```python
from build123d import *

# Parameters (mm, degrees)
F1_DEPTH = 20
F2_R     = 4
F3_DEPTH = 40.1223203436
F6_D     = 6.6


# Not quite as in the source:
# - a pattern or mirror of a feature is missing from the dataset's text; its kind, count and spacing are read off the source's solid


with BuildPart() as f1:
    # F0 (on Front) → F1 (new body, symmetric)
    with BuildSketch(Plane.XZ):
        with BuildLine():
            Line((-17.9289321881, 0), (0, 0))
            Line((0, 0), (17.9289321881, 0))
            ThreePointArc((17.9289321881, 0), (19.84234935, 0.3806023374), (21.4644660941, 1.4644660941))
            Line((21.4644660941, 1.4644660941), (55, 35))
            ThreePointArc((55, 35), (55, 39.2426406871), (50.7573593129, 39.2426406871))
            Line((50.7573593129, 39.2426406871), (18.9791847198, 7.4644660941))
            ThreePointArc((18.9791847198, 7.4644660941), (17.3570679757, 6.3806023374), (15.4436508139, 6))
            Line((15.4436508139, 6), (0, 6))
            Line((0, 6), (-15.4436508139, 6))
            ThreePointArc((-15.4436508139, 6), (-17.3570679757, 6.3806023374), (-18.9791847198, 7.4644660941))
            Line((-18.9791847198, 7.4644660941), (-50.7573593129, 39.2426406871))
            ThreePointArc((-50.7573593129, 39.2426406871), (-55, 39.2426406871), (-55, 35))
            Line((-55, 35), (-21.4644660941, 1.4644660941))
            ThreePointArc((-21.4644660941, 1.4644660941), (-19.84234935, 0.3806023374), (-17.9289321881, 0))
        make_face()
    extrude(amount=F1_DEPTH, both=True)

    # F2 (on Top) → F3 (cut, through all)
    with BuildSketch(Plane.XY):
        Circle(F2_R)
    extrude(amount=F3_DEPTH, mode=Mode.SUBTRACT)

    # F6 (through all)
    with Locations(Plane(origin=(10, 0, -10), x_dir=(0, 1, 0), z_dir=(0.7071067812, 0, -0.7071067812))):
        with Locations((0, 53.1789772213)):
            f6 = Hole(F6_D / 2)

    # F6_copies: F6 across plane
    add(f6.mirror(Plane(origin=(0, 0, 0), x_dir=(0, 0, -1), z_dir=(-1, 0, 0))), mode=Mode.SUBTRACT)


solid = f1.part
```
Build history of the part. All positions in model axes, mm. A direction names the side the tool comes from. Round coordinates to 2 decimals unless told otherwise and drop trailing zeros. Order: outer loops, then holes, each group sorted by start corner. A loop starts at its lowest first (then second) coordinate and runs counter-clockwise, first axis right, second up. Notation, with made-up numbers: (-10.5, 51.5) - (23.5, 51.5) arc R5 cw to (23.5, 57.5) - close; hole circle Ø7 at (-12.5, -31.5). An arc over 180 degrees is marked (long way). Use a Markdown table: item, result.
1) Saw through at B-B on y = 0. Write the cut outline in (x, z), and give its area (3 significant figures).
Recorded:
| item | result |
|---|---|
| outline | (-55, 35) - (-49.94, 29.94) - (-45.69, 34.18) - (-50.76, 39.24) arc R3 ccw to start; (-45.27, 25.27) - (-21.46, 1.46) arc R5 ccw to (-17.93, 0) - (-4, 0) - (-4, 6) - (-15.44, 6) arc R5 cw to (-18.98, 7.46) - (-41.03, 29.51) - close; (4, 0) - (17.93, 0) arc R5 ccw to (21.46, 1.46) - (45.27, 25.27) - (41.03, 29.51) - (18.98, 7.46) arc R5 cw to (15.44, 6) - (4, 6) - close; (45.69, 34.18) - (49.94, 29.94) - (55, 35) arc R3 ccw to (50.76, 39.24) - close |
| area | 705 mm² |
2) Saw through at C-C on y = -12. Write the cut outline in (x, z).
Recorded:
| item | result |
|---|---|
| outline | (-55, 35) - (-21.46, 1.46) arc R5 ccw to (-17.93, 0) - (17.93, 0) arc R5 ccw to (21.46, 1.46) - (55, 35) arc R3 ccw to (50.76, 39.24) - (18.98, 7.46) arc R5 cw to (15.44, 6) - (-15.44, 6) arc R5 cw to (-18.98, 7.46) - (-50.76, 39.24) arc R3 ccw to start |
3) Pull direction X, two halves, no side cores. Call faces 3 (the face through (-54.95, -0.28, 39.29)), 4 (the face through (-19.87, -0.28, 0.39)), 5 (the face through (-4.2, -0.3, 0)): pulls with the +X half, pulls with the -X half, needs draft (parallel to the pull), parting line crosses it, or undercut.
Recorded:
| item | result |
|---|---|
| face 3 | undercut |
| face 4 | pulls with the -X half |
| face 5 | needs draft |
4) Wall check: L1, parallel to Y at x = 0, z = 3.75; L2, parallel to Z at x = -9.5, y = -12; L3, parallel to X at y = 14, z = 17.5. Give the ranges that are in metal, low to high.
Recorded:
| item | result |
|---|---|
| L1 | y = -20 to -4, 4 to 20 |
| L2 | z = 0 to 6 |
| L3 | x = -37.5 to -29.01, 29.01 to 37.5 |
5) Flat gauge pins, fed straight in: pin 1 Ø1.5 at (x, z) = (-42.5, 32) entering from +Y; pin 2 Ø6.5 at (x, y) = (0, 0) entering from +Z; pin 3 Ø1.5 at (x, y) = (20.5, 7) entering from +Z; pin 4 Ø4 at (y, z) = (5, 31) entering from -X. Where does each tip first touch, or does it go through?
Recorded:
| item | result |
|---|---|
| pin 1 | stops at y = 20 |
| pin 2 | passes through |
| pin 3 | stops at z = 9.74 |
| pin 4 | stops at x = -53 |
6) Tool access for faces 1 (the face through (17.4, -0.3, 6.4)), 2 (the face through (19.82, -0.28, 0.37)): list every direction of +Z, -Z, +X, -X, +Y, -Y with a clear straight run to the whole face (end or side of a thin tool).
Recorded:
| item | result |
|---|---|
| face 1 | +Z, +Y, -Y |
| face 2 | -Z, +X, +Y, -Y |
7) Saw through at A-A on x = 0. Write the cut outline in (y, z).
Recorded:
| item | result |
|---|---|
| outline | (-20, 0) - (-4, 0) - (-4, 6) - (-20, 6) - close; (4, 0) - (20, 0) - (20, 6) - (4, 6) - close |
